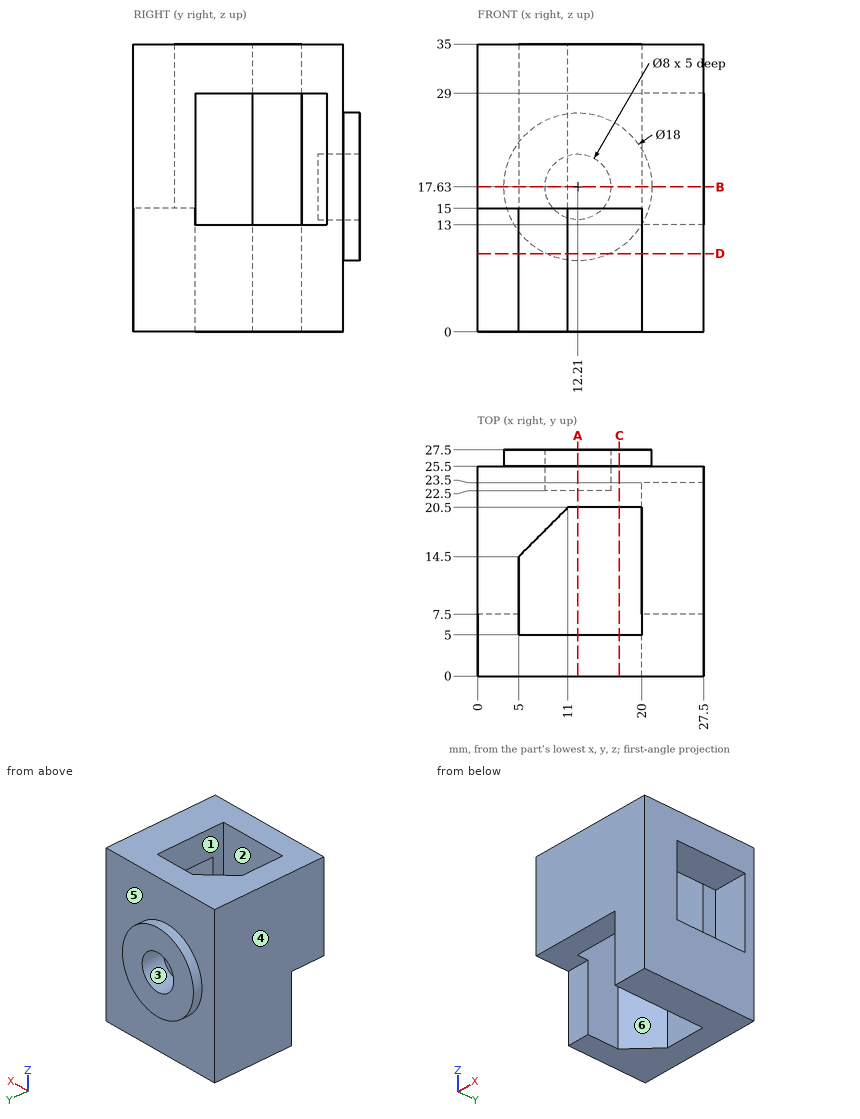
Check sheet for the drawn part. Datum: minimum x, y, z corner. Units: mm. A direction names the side the tool comes from. Round coordinates to 2 decimals unless told otherwise and drop trailing zeros. Loops run counter-clockwise (first coordinate to the right, second up) from the corner with the lowest first, then second, coordinate; pieces in that order, holes last. Notation, with made-up numbers: (16, -12.5) -> (33, -12.5) arc R27 ccw to (33, 4.5) -> close; hole circle Ø7 at (25, 10). An arc over 180 degrees is marked (long way). Put each result on its own line as item: value. Start each with the question number.
1. Gauge pin test, flat ends, axial feed: pin 1 (4 mm diameter, centred on x = 1.5, z = 5.5, fed in from -Y); pin 2 (7 mm diameter, centred on x = 12.21, z = 17.63, fed in from +Y); pin 3 (6 mm diameter, centred on x = 24.5, z = 22, fed in from +Y). Record the tip position at first contact, or that the pin passes through.
2. Section check D-D (z = 9.5). Enter the section's corners in (x, y), plus the area to 3 significant figures.
3. Access from +Z, -Z, +X, -X, +Y, -Y to the whole of each face (thin tool, end or side, straight path). Record for the marked faces 1, 2 and 3.
4. Scan lines: probe 1 along Y at (x, z) = (22, 20); probe 2 along X at (y, z) = (23.65, 17.63); probe 3 along Z at (x, y) = (12.21, 24.2). Record each from-to range of solid material in increasing order.
5. Section check C-C (x = 17.25). Enter the section's corners in (y, z).
6. Section check B-B (z = 17.63). Enter the section's corners in (x, y), plus the area to 3 significant figures.
7. Section check A-A (x = 12.21). Enter the section's corners in (y, z), plus the area to 3 significant figures.
8. Draft check along X on the marked faces 4, 5 and 6. Enter one of: +X half, -X half, draft (parallel to the pull), parting line (faces both ways), or undercut.
Findings:
1. pin 1: stops at y = 7.5
1. pin 2: stops at y = 22.5
1. pin 3: stops at y = 25.5
2. outline: (0, 7.5) -> (5, 7.5) -> (5, 14.5) -> (11, 20.5) -> (20, 20.5) -> (20, 0) -> (27.5, 0) -> (27.5, 25.5) -> (16.07, 25.5) -> (16.07, 27.5) -> (8.35, 27.5) -> (8.35, 25.5) -> (0, 25.5) -> close
2. area: 390 mm^2
3. face 1: -Z
3. face 2: +Z, -Z
3. face 3: +Y
4. probe 1: y = 0 to 7.5, 23.5 to 25.5
4. probe 2: x = 0 to 8.21, 16.21 to 27.5
4. probe 3: z = 0 to 13.63, 21.63 to 35
5. outline: (0, 15) -> (5, 15) -> (5, 35) -> (0, 35) -> close; (20.5, 0) -> (25.5, 0) -> (25.5, 10.17) -> (27.5, 10.17) -> (27.5, 25.09) -> (25.5, 25.09) -> (25.5, 35) -> (20.5, 35) -> close
6. outline: (0, 0) -> (27.5, 0) -> (27.5, 7.5) -> (20, 7.5) -> (20, 5) -> (5, 5) -> (5, 14.5) -> (11, 20.5) -> (20, 20.5) -> (20, 23.5) -> (27.5, 23.5) -> (27.5, 25.5) -> (21.21, 25.5) -> (21.21, 27.5) -> (16.21, 27.5) -> (16.21, 22.5) -> (8.21, 22.5) -> (8.21, 27.5) -> (3.21, 27.5) -> (3.21, 25.5) -> (0, 25.5) -> close
6. area: 363 mm^2
7. outline: (0, 15) -> (5, 15) -> (5, 35) -> (0, 35) -> close; (20.5, 0) -> (25.5, 0) -> (25.5, 8.63) -> (27.5, 8.63) -> (27.5, 13.63) -> (22.5, 13.63) -> (22.5, 21.63) -> (27.5, 21.63) -> (27.5, 26.63) -> (25.5, 26.63) -> (25.5, 35) -> (20.5, 35) -> close
7. area: 271 mm^2
8. face 4: -X half
8. face 5: draft
8. face 6: undercut
